Geometry check sheet. Reference: the model listing, model coordinates, mm. Give positions to 0.01 mm unless a question says otherwise; leave off trailing zeros. Write each loop counter-clockwise with the first axis right and the second up, starting at its lowest first coordinate (ties: lowest second). Pieces come first, ordered by that corner, then holes. Notation, with made-up numbers: (41.5, 25) -> (76.5, 25) arc R34 ccw to (76.5, 63) -> close; hole circle Ø4 at (67.25, 89.25). An arc over 180 degrees is marked (long way). Write item = value, one per line. Start each with the question number.
1. Cross-section at A-A, the plane x = -62.25. Record the cut outline in (y, z), plus the area to 3 significant figures.
2. Thickness scan on line 1 along X through (y, z) = (130, 1.05); line 2 along Y through (x, z) = (-122.25, 2.1); line 3 along Y through (x, z) = (-62.25, 1). Record the ranges inside material, lowest first.
3. Depth check by flat-ended pin: P1, Ø4, axis at x = -122.25, y = -130, coming from the -Z side. Enter the tip coordinate at first touch or a pass-through.
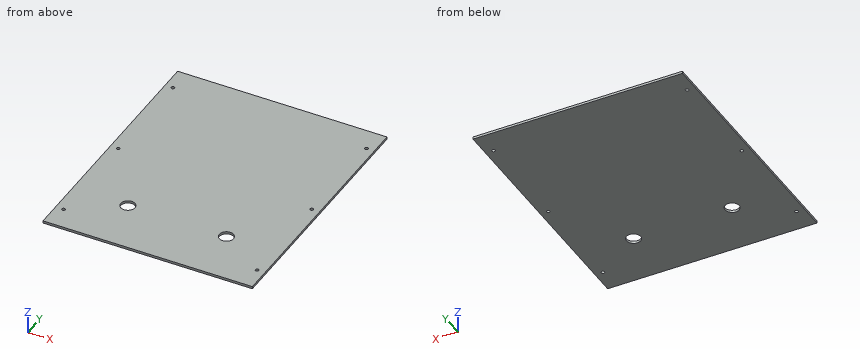
```python
from build123d import *

# Parameters (mm, degrees)
F1_W     = 264.5
F1_H     = 320
F2_DEPTH = 3
F4_D     = 4.2
F4_DEPTH = 4
F4_TIP   = 1.2618073
F5_R     = 9
F6_DEPTH = 3


# Not quite as in the source:
# - a pattern or mirror of a feature is missing from the dataset's text; its kind, count and spacing are read off the source's solid


with BuildPart() as f2:
    # F1 (on Top) → F2 (new body)
    with BuildSketch(Plane.XY):
        Rectangle(F1_W, F1_H)
    extrude(amount=F2_DEPTH)

    # F4
    with Locations(Plane.XY.offset(3)):
        with Locations((-122.25, 130), (-122.25, 0), (-122.25, -130)):
            f4 = Hole(F4_D / 2, depth=F4_DEPTH)
            with Locations((0, 0, -(F4_DEPTH + F4_TIP / 2))):  # 118° drill point
                Cone(0, F4_D / 2, F4_TIP, mode=Mode.SUBTRACT)

    # F4_copies: F4 across plane
    add(f4.mirror(Plane(origin=(0, 0, 0), x_dir=(0, 0, 1), z_dir=(1, 0, 0))), mode=Mode.SUBTRACT)

    # F5 (on face) → F6 (cut, through all)
    with BuildSketch(Plane.XY.offset(3)):
        with Locations((-62.25, -90)):
            Circle(F5_R)
        with Locations((62.25, -90)):
            Circle(F5_R)
    extrude(amount=-F6_DEPTH, mode=Mode.SUBTRACT)


solid = f2.part
```
Answers:
q1.outline = (-160, 0) -> (-99, 0) -> (-99, 3) -> (-160, 3) -> close; (-81, 0) -> (160, 0) -> (160, 3) -> (-81, 3) -> close
q1.area = 906 mm^2
q2.line_1 = -132.25 to -124.35, -120.15 to 120.15, 124.35 to 132.25
q2.line_2 = -160 to -132.1, -127.9 to -2.1, 2.1 to 127.9, 132.1 to 160
q2.line_3 = -160 to -99, -81 to 160
q3.P1 = through
